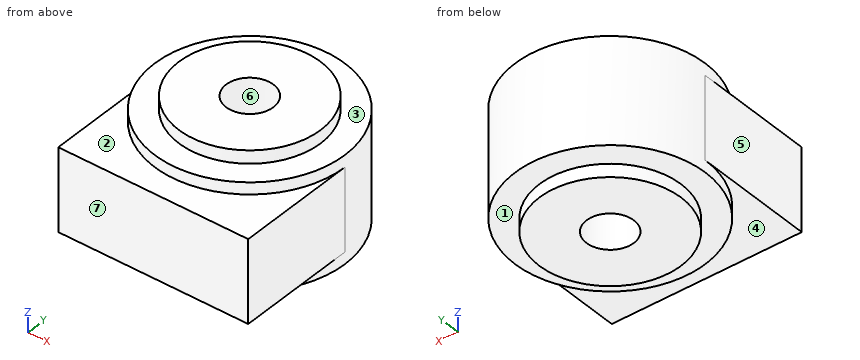
```python
from build123d import *

# Parameters (mm, degrees)
SKETCH1_W               = 80.5
SKETCH1_H               = 50.75
BOSS_EXTRUDE1_DEPTH     = 17.5
SKETCH2_R               = 40.25
BOSS_EXTRUDE2_DEPTH     = 22.5
SKETCH3_R               = 30
BOSS_EXTRUDE3_DEPTH     = 28
CUT_EXTRUDE1_DEPTH      = 104.368575979
CUT_EXTRUDE1_DEPTH_BACK = 104.368575979
SKETCH4_R               = 10


with BuildPart() as part:
    # Sketch1 → Boss-Extrude1 (new, symmetric)
    with BuildSketch(Plane.XY):
        with Locations((0, 25.375)):
            Rectangle(SKETCH1_W, SKETCH1_H)
    extrude(amount=BOSS_EXTRUDE1_DEPTH, both=True)

    # Sketch2 → Boss-Extrude2 (add, symmetric)
    with BuildSketch(Plane.XY):
        with Locations((0, 50.75)):
            Circle(SKETCH2_R)
    extrude(amount=BOSS_EXTRUDE2_DEPTH, both=True)

    # Sketch3 → Boss-Extrude3 (add, symmetric)
    with BuildSketch(Plane.XY):
        with Locations((0, 50.75)):
            Circle(SKETCH3_R)
    extrude(amount=BOSS_EXTRUDE3_DEPTH, both=True)

    # Sketch4 → Cut-Extrude1 (cut, two sides: drawn at the far end of the back side and taken through both)
    with BuildSketch(Plane.XY.offset(-CUT_EXTRUDE1_DEPTH_BACK)):
        with Locations((0, 50.75)):
            Circle(SKETCH4_R)
    extrude(amount=CUT_EXTRUDE1_DEPTH + CUT_EXTRUDE1_DEPTH_BACK, mode=Mode.SUBTRACT)


solid = part.part
```
Source: CAD feature listing. Evaluate the final solid. Frame: model axes, mm. Face numbers are marked on the shaded views. A direction names the side the tool comes from. Coordinates: 2 decimals unless noted, no trailing zeros. Loops run counter-clockwise (first coordinate to the right, second up) from the corner with the lowest first, then second, coordinate; pieces in that order, holes last. Notation, with made-up numbers: M -25.5,40 L -15.5,40 A5 cw -15.5,44 Z; hole C 67,54 d5. An arc over 180 degrees is marked long. Put each result on its own line as item: value. Start each with the question number.
1) Cut plane D-D on y = 82. Return the cut outline in (x, z).
2) Pull-direction query (Y, two-part tool) for the marked faces 5, 6 and 7; classes: pulls with the +Y half, pulls with the -Y half, needs draft (parallel to the pull), parting line crosses it, or undercut.
3) Contact query for flat-ended pins moving along their axis: pin 1 Ø2 at (x, z) = (20, -19) entering from +Y; pin 2 Ø2 at (x, y) = (31.5, 75) entering from -Z; pin 3 Ø2 at (x, y) = (7.5, 53.5) entering from +Z; pin 4 Ø12 at (y, z) = (63.5, 10) entering from +X. Output: stop coordinate, or through.
4) Cut plane A-A on x = 0. Return the cut outline in (y, z), then the cut area to 3 significant figures.
5) Cut plane C-C on x = 25.5. Return the cut outline in (y, z), then the cut area to 3 significant figures.
6) Cut plane B-B on z = -9.5. Return the cut outline in (x, y), then the cut area to 3 significant figures.
7) Ray query, L1, parallel to X at y = 50.75, z = 1.5; L2, parallel to Y at x = -0.5, z = -3.5; L3, parallel to Z at x = -9, y = 5.5. Return the intervals inside material, ascending. Write a range as from..to.
8) Reachability of the marked faces 1, 2, 3 and 4 from +Z, -Z, +X, -X, +Y, -Y: full face, straight path, thin tool, end or side. Return the list, or none.
The answers:
1. outline: M -25.37,-22.5 L 25.37,-22.5 L 25.37,22.5 L -25.37,22.5 Z
2. face 5: needs draft
2. face 6: undercut
2. face 7: pulls with the -Y half
3. pin 1: stops at y = 86.23
3. pin 2: stops at z = -22.5
3. pin 3: passes through
3. pin 4: stops at x = 39.68
4. outline: M 0,-17.5 L 10.5,-17.5 L 10.5,-22.5 L 20.75,-22.5 L 20.75,-28 L 40.75,-28 L 40.75,28 L 20.75,28 L 20.75,22.5 L 10.5,22.5 L 10.5,17.5 L 0,17.5 Z; M 60.75,-28 L 80.75,-28 L 80.75,-22.5 L 91,-22.5 L 91,22.5 L 80.75,22.5 L 80.75,28 L 60.75,28 Z
4. area: 3,530 mm²
5. outline: M 0,-17.5 L 19.61,-17.5 L 19.61,-22.5 L 34.95,-22.5 L 34.95,-28 L 66.55,-28 L 66.55,-22.5 L 81.89,-22.5 L 81.89,22.5 L 66.55,22.5 L 66.55,28 L 34.95,28 L 34.95,22.5 L 19.61,22.5 L 19.61,17.5 L 0,17.5 Z
5. area: 3,840 mm²
6. outline: M -40.25,0 L 40.25,0 L 40.25,50.75 A40.25 ccw -40.25,50.75 Z; hole C 0,50.75 d20
6. area: 6,320 mm²
7. L1: x = -40.25..-10, 10..40.25
7. L2: y = 0..40.76, 60.74..91
7. L3: z = -17.5..17.5
8. face 1: -Z
8. face 2: +Z, -Y
8. face 3: +Z
8. face 4: -Z, -Y
